Autodesk Inventor part; units mm, degrees
ref_plane "YZ Plane" through (0, 0, 0) normal (1, 0, 0) x (0, 1, 0)
ref_plane "XZ Plane" through (0, 0, 0) normal (0, 1, 0) x (-1, 0, 0)
ref_plane "XY Plane" through (0, 0, 0) normal (0, 0, 1) x (1, 0, 0)
sketch "Sketch1" plane through (0, 0, 0) normal (1, 0, 0) x (0, 1, 0)
  line L0 (0, 0) -> (101.6, 0)
  line L1 (101.6, 0) -> (101.6, 57.15)
  line L2 (0, 57.15) -> (0, 0)
  line L3 (98.425, 57.15) -> (98.425, 3.175)
  line L4 (98.425, 3.175) -> (3.175, 3.175)
  line L5 (3.175, 3.175) -> (3.175, 57.15)
  line L6 (101.6, 57.15) -> (98.425, 57.15)
  line L7 (3.175, 57.15) -> (0, 57.15)
  dimension "d0" = 101.6
  dimension "d1" = 57.15
  dimension "d2" = 3.175
extrude "Extrusion1" add sketch "Sketch1" against normal blind 2438.4
properties part number "channel2.25x4" material "Aluminum 6061"
Read the model definition and answer for the solid it produces. Units are mm, in the model's axes. A direction names the side the tool comes from. Round coordinates to 2 decimals unless told otherwise and drop trailing zeros. Write each loop counter-clockwise with the first axis right and the second up, starting at its lowest first coordinate (ties: lowest second). Pieces come first, ordered by that corner, then holes. Notation, with made-up numbers: M 13,37.25 L 26,37.25 A9 cw 26,44.25 Z; hole C -29,13 d2. An arc over 180 degrees is marked long. Use a Markdown table: item, result.
1) The part is cut by section B-B (x = -963.5). Write down the section's boundary in (y, z) (3 decimals), plus the area to 3 significant figures.
Answers follow:
| item | result |
|---|---|
| outline | M 0,0 L 101.6,0 L 101.6,57.15 L 98.425,57.15 L 98.425,3.175 L 3.175,3.175 L 3.175,57.15 L 0,57.15 Z |
| area | 665 mm2 |
2) A tool of negligible diameter and unlimited length cuts with its end or side. For faces 1 (the flat face through (-1202, 3.175, 30)), 2 (the flat face through (-1202, 101.6, 28)), from which of +Z, -Z, +X, -X, +Y, -Y can it reach the whole face along a straight path? Write none if from no direction.
Answers follow:
| item | result |
|---|---|
| face 1 | +Z, +X, -X |
| face 2 | +Z, -Z, +X, -X, +Y |
3) The part is cut by section A-A (z = 38). Write down the section's boundary in (x, y) (3 decimals).
Answers follow:
| item | result |
|---|---|
| outline | M -2438.4,0 L 0,0 L 0,3.175 L -2438.4,3.175 Z; M -2438.4,98.425 L 0,98.425 L 0,101.6 L -2438.4,101.6 Z |
4) For a pull along X with two mould halves and no side action, classify faces 3 (the flat face through (-1202, 51, 3.175)), 4 (the flat face through (-2438.4, 51, 1)), 5 (the flat face through (0, 51, 1)) as pulls with the +X half, pulls with the -X half, needs draft (parallel to the pull), parting line crosses it, or undercut.
Answers follow:
| item | result |
|---|---|
| face 3 | needs draft |
| face 4 | pulls with the -X half |
| face 5 | pulls with the +X half |
5) Flat-ended cylindrical pins translate along their axes: pin 1 (3 mm diameter, centred on x = -281.5, y = 31, fed in from -Z); pin 2 (10 mm diameter, centred on x = -1377, y = 60, fed in from +Z) (3 decimals). Find the tip coordinate at first contact, or state that the pin passes through.
Answers follow:
| item | result |
|---|---|
| pin 1 | stops at z = 0 |
| pin 2 | stops at z = 3.175 |
6) The part is cut by section C-C (y = 74). Write down the section's boundary in (x, z) (3 decimals).
Answers follow:
| item | result |
|---|---|
| outline | M -2438.4,0 L 0,0 L 0,3.175 L -2438.4,3.175 Z |
7) Straight lines are drawn through the part: line 1 along Y through (x, z) = (-318.5, 12) (3 decimals); line 2 along Z through (x, y) = (-1416, 59.5) (3 decimals). For each, find the intervals that lie inside material, in ascending order. Write a range as [from, to].
Answers follow:
| item | result |
|---|---|
| line 1 | y = [0, 3.175], [98.425, 101.6] |
| line 2 | z = [0, 3.175] |
